Here's the drawing with two shaded views (mm, measured from the low corner). I have some questions. A direction names the side the tool comes from. Give positions to 0.01 mm unless a question says otherwise; leave off trailing zeros. Loops run counter-clockwise (first coordinate to the right, second up) from the corner with the lowest first, then second, coordinate; pieces in that order, holes last. Notation, with made-up numbers: (37, 1) - (85, 1) arc R9 cw to (85, 16) - close; hole circle Ø6 at (-7.5, 29.5). An arc over 180 degrees is marked (long way). Answer as a JSON object with one key per item and string values. Group by question number.
Item 1: Suppose I cut it at A-A on x = 12. Write out the boundary of the cut face in (y, z).
Item 2: Suppose I cut it at D-D on x = 2.5. Write out the boundary of the cut face in (y, z).
Item 3: Please list where these lines run through material, in increasing order: L1, parallel to X at y = 5.25, z = 2.5 (1 decimal); L2, parallel to Z at x = 15.5, y = 1.5; L3, parallel to X at y = 1.5, z = 16.
Item 4: Which directions (+Z, -Z, +X, -X, +Y, -Y) give clear straight access to the entire face, cutting with the end or side of a thin tool? Please do the marked faces 4, 5, 6, 7 and 8.
Item 5: Suppose I cut it at B-B on z = 14.75. Write out the boundary of the cut face in (x, y).
Item 6: Suppose I cut it at C-C on y = 2. Write out the boundary of the cut face in (x, z) (1 decimal), and give its area (3 significant figures).
Item 7: Will these pins go through, and if not, where does the flat tip stop? pin 1 (2 mm diameter, centred on y = 2, z = 1, fed in from -X); pin 2 (3 mm diameter, centred on x = 27, y = 4.5, fed in from -Z); pin 3 (2 mm diameter, centred on x = 15, y = 2, fed in from -Z).
Item 8: Thinking about a two-plate mould opening in Z: for the marked faces 1, 2 and 3, which applies, pulls with the +Z half, pulls with the -Z half, needs draft (parallel to the pull), parting line crosses it, or undercut?
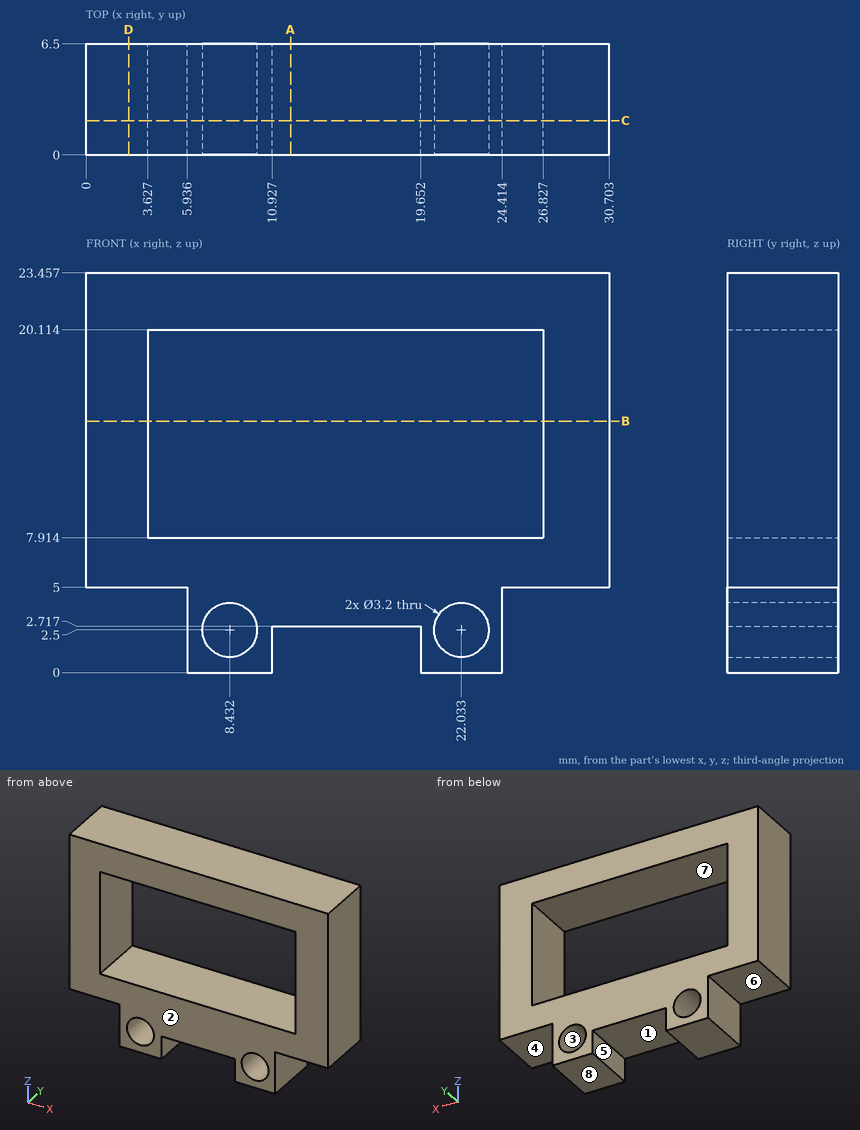
Worked out:
{
 "1": {"outline": "(0, 2.72) - (6.5, 2.72) - (6.5, 7.91) - (0, 7.91) - close; (0, 20.11) - (6.5, 20.11) - (6.5, 23.46) - (0, 23.46) - close"},
 "2": {"outline": "(0, 5) - (6.5, 5) - (6.5, 23.46) - (0, 23.46) - close"},
 "3": {"L1": "x = 5.9 to 6.8, 10 to 10.9, 19.7 to 20.4, 23.6 to 24.4", "L2": "z = 2.72 to 7.91, 20.11 to 23.46", "L3": "x = 0 to 3.63, 26.83 to 30.7"},
 "4": {"face 4": "-Z, +X, +Y, -Y", "face 5": "-Z, +Y, -Y", "face 6": "-Z, -X, +Y, -Y", "face 7": "+Y, -Y", "face 8": "-Z, +X, -X, +Y, -Y"},
 "5": {"outline": "(0, 0) - (3.63, 0) - (3.63, 6.5) - (0, 6.5) - close; (26.83, 0) - (30.7, 0) - (30.7, 6.5) - (26.83, 6.5) - close"},
 "6": {"outline": "(0, 5) - (5.9, 5) - (5.9, 0) - (10.9, 0) - (10.9, 2.7) - (19.7, 2.7) - (19.7, 0) - (24.4, 0) - (24.4, 5) - (30.7, 5) - (30.7, 23.5) - (0, 23.5) - close; hole (3.6, 7.9) - (26.8, 7.9) - (26.8, 20.1) - (3.6, 20.1) - close; hole circle Ø3.2 at (8.4, 2.5); hole circle Ø3.2 at (22, 2.5)", "area": "336 mm2"},
 "7": {"pin 1": "stops at x = 5.94", "pin 2": "stops at z = 5", "pin 3": "stops at z = 2.72"},
 "8": {"face 1": "pulls with the -Z half", "face 2": "needs draft", "face 3": "undercut"}
}
